```python
from build123d import *

# Parameters (mm, degrees)
SKETCH_3_W      = 38.5
SKETCH_3_H      = 34
SKETCH_3_R      = 3
EXTRUDE_1_DEPTH = 2
SKETCH_4_R      = 12
EXTRUDE_3_DEPTH = 4
SKETCH_6_R      = 4.758056851
EXTRUDE_4_DEPTH = 6


with BuildPart() as part:
    # 草图3 → 凸台-拉伸1 (new body)
    with BuildSketch(Plane(origin=(0, 0, 0), x_dir=(1, 0, 0), z_dir=(0, 1, 0))):
        with Locations((-10.049882631, -25.638405163)):
            Rectangle(SKETCH_3_W, SKETCH_3_H)
        with Locations(Location((-24.299882631, -13.638405163, 0), (0, 0, 270))):
            Circle(SKETCH_3_R, mode=Mode.SUBTRACT)
        with Locations(Location((4.200117369, -13.638405163, 0), (0, 0, 270))):
            Circle(SKETCH_3_R, mode=Mode.SUBTRACT)
        with Locations(Location((-24.299882631, -37.638405163, 0), (0, 0, 270))):
            Circle(SKETCH_3_R, mode=Mode.SUBTRACT)
        with Locations(Location((4.200117369, -37.638405163, 0), (0, 0, 270))):
            Circle(SKETCH_3_R, mode=Mode.SUBTRACT)
    extrude(amount=EXTRUDE_1_DEPTH)

    # 草图4 → 凸台-拉伸3 (add)
    with BuildSketch(Plane(origin=(0, 0, 0), x_dir=(1, 0, 0), z_dir=(0, 1, 0))):
        with Locations(Location((-10.049882631, -25.638405163, 0), (0, 0, 270))):
            Circle(SKETCH_4_R)
    extrude(amount=EXTRUDE_3_DEPTH)

    # 草图6 → 凸台-拉伸4 (add)
    with BuildSketch(Plane(origin=(0, 0, 0), x_dir=(1, 0, 0), z_dir=(0, 1, 0))):
        with Locations(Location((-10.049882631, -25.638405163, 0), (0, 0, 270))):
            Circle(SKETCH_6_R)
    extrude(amount=EXTRUDE_4_DEPTH)


solid = part.part
```
Design review of the part built by this model. Coordinates are the model's own, in mm. A direction names the side the tool comes from. Round coordinates to 2 decimals unless told otherwise and drop trailing zeros. Order: outer loops, then holes, each group sorted by start corner. A loop starts at its lowest first (then second) coordinate and runs counter-clockwise, first axis right, second up. Notation, with made-up numbers: (-11, -31.5) - (17, -31.5) arc R27 ccw to (17, 4.5) - close; hole circle Ø8 at (-35, 68.25). An arc over 180 degrees is marked (long way). Return JSON: item names as keys, results as strings.
Q1. Consider section C-C on z = 27.5. Write out the cut boundary in (x, y).
Computed values:
{"outline": "(-29.3, 0) - (9.2, 0) - (9.2, 2) - (1.8, 2) - (1.8, 4) - (-5.67, 4) - (-5.67, 6) - (-14.43, 6) - (-14.43, 4) - (-21.9, 4) - (-21.9, 2) - (-29.3, 2) - close"}
Q2. Consider section D-D on x = -20. Write out the cut boundary in (y, z), plus the area to 3 significant figures.
Computed values:
{"outline": "(0, 8.64) - (2, 8.64) - (2, 18.93) - (4, 18.93) - (4, 32.35) - (2, 32.35) - (2, 42.64) - (0, 42.64) - close", "area": "94.8 mm2"}
Q3. The part is to be moulded in two halves that separate along X. For faces 1 (the cylindrical face through (-11.872, 4.986, 30.034)), 2 (the cylindrical face through (-23.4, 1, 40.5)), 3 (the cylindrical face through (5.1, 1, 40.5)), 4 (the flat face through (-15, 4, 25)), say which applies: pulls with the +X half, pulls with the -X half, needs draft (parallel to the pull), parting line crosses it, or undercut.
Computed values:
{"face 1": "parting line crosses it", "face 2": "undercut", "face 3": "undercut", "face 4": "needs draft"}
Q4. Consider section A-A on z = 38.5. Write out the cut boundary in (x, y), plus the area to 3 significant figures.
Computed values:
{"outline": "(-29.3, 0) - (-27.17, 0) - (-27.17, 2) - (-29.3, 2) - close; (-21.43, 0) - (1.33, 0) - (1.33, 2) - (-21.43, 2) - close; (7.07, 0) - (9.2, 0) - (9.2, 2) - (7.07, 2) - close", "area": "54.0 mm2"}
Q5. Consider section B-B on x = 3. Write out the cut boundary in (y, z), plus the area to 3 significant figures.
Computed values:
{"outline": "(0, 8.64) - (2, 8.64) - (2, 10.89) - (0, 10.89) - close; (0, 16.39) - (2, 16.39) - (2, 34.89) - (0, 34.89) - close; (0, 40.39) - (2, 40.39) - (2, 42.64) - (0, 42.64) - close", "area": "46.0 mm2"}
Q6. Machinability: for faces 5 (the cylindrical face through (-21.765, 2.986, 23.037)), 6 (the flat face through (-10, 0, 25)), which of the approach directions +Z, -Z, +X, -X, +Y, -Y give a long, thin tool a straight path to every point of the face, cutting with its end or side? Answer none if there is none.
Computed values:
{"face 5": "+Y", "face 6": "+Z, -Z, +X, -X, -Y"}
Q7. Wall thickness on L1, parallel to X at y = 1.5, z = 15.5; L2, parallel to X at y = 0.8, z = 39; L3, parallel to Y at x = -17, z = 29.5: over which ranges is each line inside the solid? List them lowest first. Write a range as [from, to].
Computed values:
{"L1": "x = [-29.3, -26.65], [-21.95, 1.85], [6.55, 9.2]", "L2": "x = [-29.3, -26.97], [-21.63, 1.53], [6.87, 9.2]", "L3": "y = [0, 4]"}
Q8. For pin 1 Ø6 at (x, z) = (-7.5, 33) entering from +Y; pin 2 Ø3 at (y, z) = (4, 23.5) entering from -X; pin 3 Ø10 at (x, z) = (-15.5, 28) entering from +Y; pin 4 Ø5 at (x, z) = (4.2, 37.64) entering from -Y, all flat-tipped, find the tip position at first contact; note any pin that passes through.
Computed values:
{"pin 1": "stops at y = 4", "pin 2": "stops at x = -22.03", "pin 3": "stops at y = 6", "pin 4": "passes through"}
